from build123d import *

# Parameters (mm, degrees)
F1_DEPTH  = 60
F3_DEPTH  = 5
F6_DEPTH  = 5
F7_R      = 4.25
F8_DEPTH  = 25
F9_R      = 3.25
F10_DEPTH = 25


with BuildPart() as f1:
    # F0 (on Right) → F1 (new body)
    with BuildSketch(Plane.YZ):
        Polygon((0, 60), (0, 0), (75, 0), (75, 5), (5, 5), (5, 60), align=None)
    extrude(amount=-F1_DEPTH)

    # F2 (on Right) → F3 (join)
    with BuildSketch(Plane.YZ):
        Polygon((75, 5), (5, 60), (5, 5), align=None)
    extrude(amount=-F3_DEPTH)

    # F5 (on offset) → F6 (join)
    with BuildSketch(Plane.YZ.offset(-60)):
        Polygon((75, 5), (5, 60), (5, 5), align=None)
    extrude(amount=F6_DEPTH)

    # F7 (on face) → F8 (cut)
    with BuildSketch(Plane.XY.offset(5)):
        with Locations((-15, 35)):
            Circle(F7_R)
        with Locations((-15, 65)):
            Circle(F7_R)
        with Locations((-45, 65)):
            Circle(F7_R)
        with Locations((-45, 35)):
            Circle(F7_R)
    extrude(amount=-F8_DEPTH, mode=Mode.SUBTRACT)

    # F9 (on face) → F10 (cut)
    with BuildSketch(Plane(origin=(0, 5, 0), x_dir=(-1, 0, 0), z_dir=(0, 1, 0))):
        with Locations((45, 20)):
            Circle(F9_R)
        with Locations((45, 50)):
            Circle(F9_R)
        with Locations((15, 50)):
            Circle(F9_R)
        with Locations((15, 20)):
            Circle(F9_R)
    extrude(amount=-F10_DEPTH, mode=Mode.SUBTRACT)


solid = f1.part
Geometry: final body of the model. Coordinates: model frame, mm. A direction names the side the tool comes from. Give positions to 0.01 mm unless a question says otherwise; leave off trailing zeros. Write each loop counter-clockwise with the first axis right and the second up, starting at its lowest first coordinate (ties: lowest second). Pieces come first, ordered by that corner, then holes.
(1) Cut plane C-C, the plane y = 35. Return loops of the section in (x, z), then the cut area to 3 significant figures.
(2) Ray query, line 1 (Z direction, x = -45, y = 1); line 2 (Y direction, x = -15, z = 1.95); line 3 (X direction, y = 27, z = 9). Return the intervals inside material, ascending.
(3) Cut plane A-A, the plane x = -45. Return loops of the section in (y, z), then the cut area to 3 significant figures.
(4) Cut plane B-B, the plane z = 50. Return loops of the section in (x, y).
(5) Access query for faces 4 (the flat face through (-55, 24, 21)), 5 (the cylindrical face through (-48.37, 62.41, 2.54)). Directions: +Z, -Z, +X, -X, +Y, -Y. A direction counts if a zero-diameter tool reaches every point of the face in a straight line with its end or side. Return the directions, or none.
(6) Mould query, pull axis Z, two halves, no side actions, for faces 1 (the flat face through (-30, 40, 5)), 2 (the flat face through (-5, 24, 21)), 3 (the cylindrical face through (-12.421, 2.535, 18.022)). Classes: released by +Z, released by -Z, zero draft, split by the parting line, or undercut.
(7) First-contact query: P1, Ø25, axis at x = -41.5, z = 42, coming from the +Y side; P2, Ø12, axis at x = -7.5, y = 55, coming from the +Z side; P3, Ø5, axis at x = -15, z = 20, coming from the +Y side; P4, Ø10, axis at x = -15, y = 35, coming from the +Z side. Flat tips, straight axial feed; report the tip coordinate or a pass-through.
(8) Cut plane D-D, the plane x = -32.5. Return loops of the section in (y, z).
Values follow:
1. outline: (-60, 0) - (-49.25, 0) - (-49.25, 5) - (-55, 5) - (-55, 36.43) - (-60, 36.43) - close; (-40.75, 0) - (-19.25, 0) - (-19.25, 5) - (-40.75, 5) - close; (-10.75, 0) - (0, 0) - (0, 36.43) - (-5, 36.43) - (-5, 5) - (-10.75, 5) - close
1. area: 529 mm2
2. line 1: z = 0 to 16.75, 23.25 to 46.75, 53.25 to 60
2. line 2: y = 0 to 30.75, 39.25 to 60.75, 69.25 to 75
2. line 3: x = -60 to -55, -5 to 0
3. outline: (0, 0) - (30.75, 0) - (30.75, 5) - (5, 5) - (5, 16.75) - (0, 16.75) - close; (0, 23.25) - (5, 23.25) - (5, 46.75) - (0, 46.75) - close; (0, 53.25) - (5, 53.25) - (5, 60) - (0, 60) - close; (39.25, 0) - (60.75, 0) - (60.75, 5) - (39.25, 5) - close; (69.25, 0) - (75, 0) - (75, 5) - (69.25, 5) - close
3. area: 500 mm2
4. outline: (-60, 0) - (-48.25, 0) - (-48.25, 5) - (-55, 5) - (-55, 17.73) - (-60, 17.73) - close; (-41.75, 0) - (-18.25, 0) - (-18.25, 5) - (-41.75, 5) - close; (-11.75, 0) - (0, 0) - (0, 17.73) - (-5, 17.73) - (-5, 5) - (-11.75, 5) - close
5. face 4: +Z, +Y
5. face 5: +Z, -Z
6. face 1: released by +Z
6. face 2: zero draft
6. face 3: undercut
7. P1: stops at y = 5
7. P2: stops at z = 25
7. P3: passes through
7. P4: stops at z = 5
8. outline: (0, 0) - (75, 0) - (75, 5) - (5, 5) - (5, 60) - (0, 60) - close
